Build history of the part. All positions in model axes, mm. A direction names the side the tool comes from. Coordinates: 2 decimals unless noted, no trailing zeros. Loops run counter-clockwise (first coordinate to the right, second up) from the corner with the lowest first, then second, coordinate; pieces in that order, holes last.
Item 1: Drill centre lines: line 1 along X through (y, z) = (4.75, 3.25); line 2 along Y through (x, z) = (9.5, 4.25); line 3 along Z through (x, y) = (30.5, 12.75). Where is each one in solid material? Low to high.
Item 2: Cut at A-A (x = 20). List the corners of the cut face in (y, z), and give its area (3 significant figures).
Item 3: Cut at D-D (y = 2.75). List the corners of the cut face in (x, z).
Item 4: Cut at B-B (y = 11.9). List the corners of the cut face in (x, z).
Item 5: Mould opens along X. For faces 1 (the face through (2.61, 13.924, 10.389)), 2 (the face through (31.8, 8, 5)), 3 (the face through (4, 12, 11.4)), 4 (the face through (30.6, 8, 4)) say: released by +X, released by -X, zero draft, split by the parting line, or undercut.
Item 6: Flat gauge pin, fed straight in: pin 1 (4.5 mm diameter, centred on x = 16.5, y = 11, fed in from +Z). Where does the tip first touch, or does it go through?
Item 7: Cut at C-C (z = 3.75). List the corners of the cut face in (x, y), and give its area (3 significant figures).
Item 8: 3-axis set-ups, long thin cutter, end or side, ignore diameter. For faces 5 (the face through (16, 15.8, 5)), 6 (the face through (16, 8, 8.4)): which of +Z, -Z, +X, -X, +Y, -Y reach the whole face in a straight line?
Autodesk Fusion 360 part; units mm, degrees
sketch "Sketch1" plane through (0, 0, 0) normal (0, 0, 1) x (1, 0, 0)
  line L0 (0, 0) -> (31.8, 0)
  line L1 (31.8, 0) -> (31.8, 15.8)
  line L2 (31.8, 15.8) -> (0, 15.8)
  line L3 (0, 15.8) -> (0, 0)
  dimension "d3" = 31.8
  dimension "d4" = 15.8
extrude "Extrude1" add sketch "Sketch1" along normal blind 9.6
shell "Shell1" thickness 1.2 removed faces 1 at (21.2, 5.2667, 0)
sketch "Sketch2" plane through (0, 0, 9.6) normal (0, 0, 1) x (-1, 0, 0)
  line L0 (0, -15.8) -> (0, 0)
  line L1 (0, 0) -> (-31.8, 0)
  line L2 (-31.8, 0) -> (-31.8, -15.8)
  line L3 (-31.8, -15.8) -> (0, -15.8)
  circle A0 centre (-3.9, -11.9) radius 2.4
  dimension "d8" = 4.8
  dimension "d9" = 3.9
  dimension "d10" = 3.9
extrude "Extrude2" add sketch "Sketch2" along normal blind 1.8 contours A0
fillet "Fillet1" radius 0.2 1 edges at (6.1376, 12.7679, 11.4)
equation "d3 = ( 3.9 * 2 ) * 1 mm + ( 8.0 * ( n_orizzontale - 1 ) ) * 1 mm"
equation "d4 = ( 3.9 * 2 ) * 1 mm + ( 8.0 * ( n_verticale - 1 ) ) * 1 mm"
Filled sheet:
1. line 1: x = 0 to 1.2, 30.6 to 31.8
1. line 2: y = 0 to 1.2, 14.6 to 15.8
1. line 3: z = 8.4 to 9.6
2. outline: (0, 0) - (1.2, 0) - (1.2, 8.4) - (14.6, 8.4) - (14.6, 0) - (15.8, 0) - (15.8, 9.6) - (0, 9.6) - close
2. area: 39.1 mm2
3. outline: (0, 0) - (1.2, 0) - (1.2, 8.4) - (30.6, 8.4) - (30.6, 0) - (31.8, 0) - (31.8, 9.6) - (0, 9.6) - close
4. outline: (0, 0) - (1.2, 0) - (1.2, 8.4) - (30.6, 8.4) - (30.6, 0) - (31.8, 0) - (31.8, 9.6) - (6.3, 9.6) - (6.3, 11.2) arc R0.2 ccw to (6.1, 11.4) - (1.7, 11.4) arc R0.2 ccw to (1.5, 11.2) - (1.5, 9.6) - (0, 9.6) - close
5. face 1: split by the parting line
5. face 2: released by +X
5. face 3: zero draft
5. face 4: undercut
6. pin 1: stops at z = 9.6
7. outline: (0, 0) - (31.8, 0) - (31.8, 15.8) - (0, 15.8) - close; hole (1.2, 1.2) - (30.6, 1.2) - (30.6, 14.6) - (1.2, 14.6) - close
7. area: 108 mm2
8. face 5: +Z, -Z, +X, -X, +Y
8. face 6: -Z
